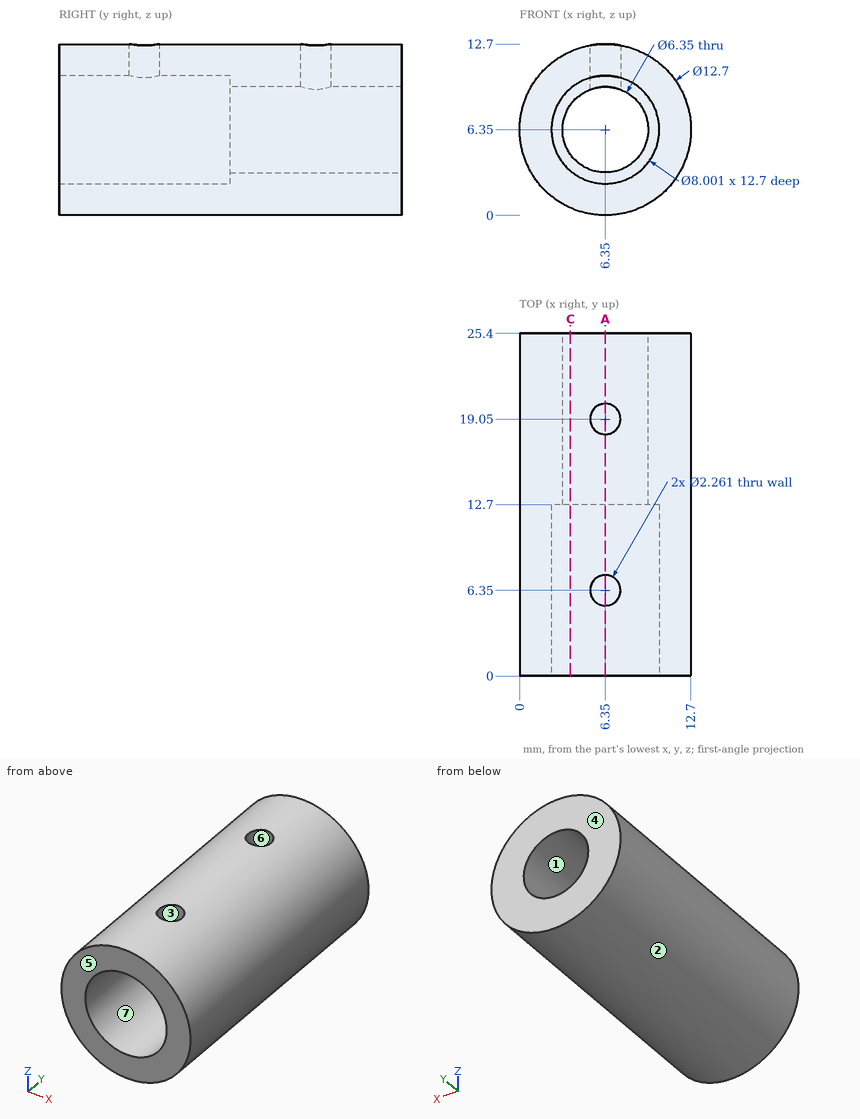
Study the drawing (mm; zero at the part's minimum x, y, z) and answer. A direction names the side the tool comes from. Round coordinates to 2 decimals unless told otherwise and drop trailing zeros. Write each loop counter-clockwise with the first axis right and the second up, starting at its lowest first coordinate (ties: lowest second). Pieces come first, ordered by that corner, then holes. Notation, with made-up numbers: (88.5, -30.75) -> (106.5, -30.75) arc R10 ccw to (106.5, -18.75) -> close; hole circle Ø11 at (49, 37.25). An arc over 180 degrees is marked (long way). Answer as CSV lines item,"result". Start each with the question number.
(1) Each of these flat-tipped pins is pushed along its axis until it touches: pin 1 (1.5 mm diameter, centred on y = 4, z = 10, fed in from -X); pin 2 (1.5 mm diameter, centred on x = 7.5, y = 5.5, fed in from +Z); pin 3 (2 mm diameter, centred on x = 6.35, y = 6.35, fed in from +Z). Where does it stop, or does it pass through?
(2) The part is cut by section C-C, the plane x = 3.75. Give the vertices of the cut face in (y, z).
(3) Find the intervals of material crossed by probe 1 along X at (y, z) = (8, 6.35); probe 2 along X at (y, z) = (16, 6.25); probe 3 along Y at (x, z) = (8, 2.75), in increasing order.
(4) The mould has two halves that part along X. Classify the marked faces 1, 2, 3 and 4: +X half, -X half, draft (parallel to the pull), parting line (faces both ways), or undercut.
(5) The part is cut by section A-A, the plane x = 6.35. Give the number of separate pieces and of enclosed holes in the cut face, then the cut area to 3 significant figures.
(6) A tool of negligible diameter and unlimited length cuts with its end or side. For the marked faces 5, 6 and 7, from which of +Z, -Z, +X, -X, +Y, -Y can it reach the whole face along a straight path? Write none if from no direction.
Output values:
1,pin 1,"stops at x = 0.7"
1,pin 2,"stops at z = 12.69"
1,pin 3,"stops at z = 2.48"
2,outline,"(0, 0.56) -> (25.4, 0.56) -> (25.4, 4.53) -> (12.7, 4.53) -> (12.7, 3.31) -> (0, 3.31) -> close; (0, 9.39) -> (12.7, 9.39) -> (12.7, 8.17) -> (25.4, 8.17) -> (25.4, 12.14) -> (0, 12.14) -> close"
3,probe 1,"x = 0 to 2.35, 10.35 to 12.7"
3,probe 2,"x = 0 to 3.18, 9.52 to 12.7"
3,probe 3,"y = 12.7 to 25.4"
4,face 1,"undercut"
4,face 2,"parting line"
4,face 3,"undercut"
4,face 4,"draft"
5,separate pieces,"4"
5,enclosed holes,"0"
5,area,"128 mm²"
6,face 5,"+Z, -Z, +X, -X, -Y"
6,face 6,"+Z"
6,face 7,"-Y"
